```python
from build123d import *

# Parameters (mm, degrees)
SKETCH1_R           = 5
BOSS_EXTRUDE1_DEPTH = 5
CUT_EXTRUDE1_DEPTH  = 6


with BuildPart() as part:
    # Sketch1 → Boss-Extrude1 (new, symmetric)
    with BuildSketch(Plane.XY):
        with BuildLine():
            Line((-94.5, 8), (94.5, 8))
            ThreePointArc((94.5, 8), (102.5, 0), (94.5, -8))
            Line((94.5, -8), (-94.5, -8))
            ThreePointArc((-94.5, -8), (-102.5, 0), (-94.5, 8))
        make_face()
        with Locations((-94.5, 0)):
            Circle(SKETCH1_R, mode=Mode.SUBTRACT)
        with Locations(Location((94.5, 0, 0), (0, 0, 180))):
            Circle(SKETCH1_R, mode=Mode.SUBTRACT)
    extrude(amount=BOSS_EXTRUDE1_DEPTH, both=True)

    # Sketch2 → Cut-Extrude1 (cut)
    with BuildSketch(Plane(origin=(0, 0, -5), x_dir=(-1, 0, 0), z_dir=(0, 0, -1))):
        with BuildLine():
            Line((-74.5, 4), (74.5, 4))
            ThreePointArc((74.5, 4), (78.5, 0), (74.5, -4))
            Line((74.5, -4), (-74.5, -4))
            ThreePointArc((-74.5, -4), (-78.5, 0), (-74.5, 4))
        make_face()
    extrude(amount=-CUT_EXTRUDE1_DEPTH, mode=Mode.SUBTRACT)


solid = part.part
```
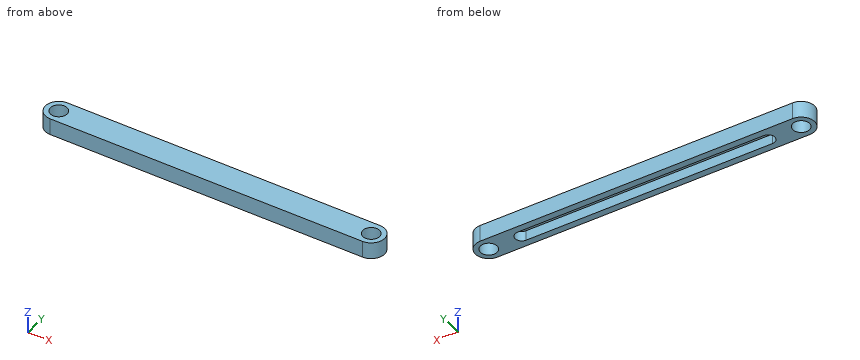
Design review of the part built by this model. Coordinates are the model's own, in mm. Give positions to 0.01 mm unless a question says otherwise; leave off trailing zeros. Loops run counter-clockwise (first coordinate to the right, second up) from the corner with the lowest first, then second, coordinate; pieces in that order, holes last. Notation, with made-up numbers: M 6.5,-10.5 L 38.5,-10.5 A24 ccw 38.5,10.5 Z; hole C 56,0 d1. An arc over 180 degrees is marked long. Return JSON: item names as keys, results as strings. Group by question number.
Item 1: We need section B-B (y = 0). Give the boundary of the cut face in (x, z), and give its area (3 significant figures).
Item 2: We need section A-A (z = -0.5). Give the boundary of the cut face in (x, y).
Item 3: Insertion check: pin 1 Ø6.5 at (x, y) = (20, 0.5) entering from -Z; pin 2 Ø1 at (y, z) = (6, -1) entering from -X. Each pin has a flat end and moves straight along its axis. Give the tip position at first contact, or say it passes through.
Item 4: For probe 1 along X at (y, z) = (1.5, 4); probe 2 along Y at (x, z) = (-94.5, 1.5); probe 3 along X at (y, z) = (3.5, 2.5), list the stretches that pass through material, from the lowest coordinate up.
Item 5: We need section C-C (x = -48.5). Give the boundary of the cut face in (y, z), and give its area (3 significant figures).
Output:
{
 "1": {"outline": "M -102.5,-5 L -99.5,-5 L -99.5,5 L -102.5,5 Z; M -89.5,-5 L -78.5,-5 L -78.5,1 L 78.5,1 L 78.5,-5 L 89.5,-5 L 89.5,5 L -89.5,5 Z; M 99.5,-5 L 102.5,-5 L 102.5,5 L 99.5,5 Z", "area": "908 mm^2"},
 "2": {"outline": "M -94.5,-8 L 94.5,-8 A8 ccw 94.5,8 L -94.5,8 A8 ccw Z; hole C -94.5,0 d10; hole M -74.5,-4 L 74.5,-4 A4 ccw 74.5,4 L -74.5,4 A4 ccw Z; hole C 94.5,0 d10"},
 "3": {"pin 1": "stops at z = 1", "pin 2": "stops at x = -100.31"},
 "4": {"probe 1": "x = -102.36 to -99.27, -89.73 to 89.73, 99.27 to 102.36", "probe 2": "y = -8 to -5, 5 to 8", "probe 3": "x = -101.69 to -98.07, -90.93 to 90.93, 98.07 to 101.69"},
 "5": {"outline": "M -8,-5 L -4,-5 L -4,1 L 4,1 L 4,-5 L 8,-5 L 8,5 L -8,5 Z", "area": "112 mm^2"}
}
